Could you check a few things on this model? Use its own coordinates, in mm. A direction names the side the tool comes from. Give positions to 0.01 mm unless a question says otherwise; leave off trailing zeros. Loops run counter-clockwise (first coordinate to the right, second up) from the corner with the lowest first, then second, coordinate; pieces in that order, holes last. Notation, with made-up numbers: M -28.75,53.5 L 30.25,53.5 A21 ccw 30.25,87.5 Z; hole C 67.5,-13 d1. An arc over 180 degrees is marked long. Answer in a Markdown table with one row per item. Add a question column.
1. Thinking about a two-plate mould opening in Z: for faces 3 (the conical face through (-0.41, 22.857, 0.17)), 4 (the cylindrical face through (3.86, 92.6, 5.04)), 5 (the flat face through (-2, 187.82, 2)), 6 (the cylindrical face through (2.435, 11.466, -0.767)), which applies, released by +Z, released by -Z, zero draft, split by the parting line, or undercut?
2. I need wall thicknesses on line 1 along X through (y, z) = (101, -0.5); line 2 along Z through (x, y) = (-3.5, 45); line 3 along Z through (x, y) = (-0.75, 164.5). Which ranges of each line are inside material? Lowest first, please. Write a range as from..to.
3. Which directions (+Z, -Z, +X, -X, +Y, -Y) give clear straight access to the entire face, cutting with the end or side of a thin tool? Please do faces 1 (the flat face through (3, 0, -3)), 2 (the cylindrical face through (1.216, 178.676, -1.115)).
4. I'm going to push flat-ended pins straight in: pin 1 Ø3 at (x, y) = (-2, 79) entering from -Z; pin 2 Ø4 at (y, z) = (150, 2.5) entering from -X; pin 3 Ø4 at (x, z) = (0, 0) entering from -Y. Where does each tip first touch, or does it pass through?
5. If we section it at B-B on y = 155.5: List the corners of the cut face in (x, z) for me.
6. If we section it at A-A on y = 13: List the corners of the cut face in (x, z) for me, then the cut area to 3 significant figures.
```python
from build123d import *

# Parameters (mm, degrees)
SKETCH1_R                         = 6.35
BOSS_EXTRUDE1_DEPTH               = 187.8203
F_1_4_20_TAPPED_HOLE1_D           = 5.1054
F_1_4_20_TAPPED_HOLE1_DEPTH       = 21.59
F_1_4_20_TAPPED_HOLE1_CSINK_D     = 7.62
F_1_4_20_TAPPED_HOLE1_CSINK_ANGLE = 100
F_1_4_20_TAPPED_HOLE1_TIP         = 1.533816902
M4X0_7_TAPPED_HOLE1_D             = 3.3
M4X0_7_TAPPED_HOLE1_DEPTH         = 17.7292
M4X0_7_TAPPED_HOLE1_CSINK_D       = 4.05
M4X0_7_TAPPED_HOLE1_CSINK_ANGLE   = 100
M4X0_7_TAPPED_HOLE1_TIP           = 0.991420021


with BuildPart() as part:
    # Sketch1 → Boss-Extrude1 (new body)
    with BuildSketch(Plane(origin=(0, 0, 0), x_dir=(1, 0, 0), z_dir=(0, 1, 0))):
        with Locations(Location((0, 0, 0), (0, 0, 90))):
            Circle(SKETCH1_R)
    extrude(amount=BOSS_EXTRUDE1_DEPTH)

    # 1/4-20 Tapped Hole1
    with Locations(Plane(origin=(0, 0, 0), x_dir=(-1, 0, 0), z_dir=(0, -1, 0))):
        with Locations((0, 0)):
            CounterSinkHole(F_1_4_20_TAPPED_HOLE1_D / 2, F_1_4_20_TAPPED_HOLE1_CSINK_D / 2, depth=F_1_4_20_TAPPED_HOLE1_DEPTH, counter_sink_angle=F_1_4_20_TAPPED_HOLE1_CSINK_ANGLE)
            with Locations((0, 0, -(F_1_4_20_TAPPED_HOLE1_DEPTH + F_1_4_20_TAPPED_HOLE1_TIP / 2))):  # 118° drill point
                Cone(0, F_1_4_20_TAPPED_HOLE1_D / 2, F_1_4_20_TAPPED_HOLE1_TIP, mode=Mode.SUBTRACT)

    # M4x0.7 Tapped Hole1
    with Locations(Plane(origin=(0, 187.8203, 0), x_dir=(1, 0, 0), z_dir=(0, 1, 0))):
        with Locations((0, 0)):
            CounterSinkHole(M4X0_7_TAPPED_HOLE1_D / 2, M4X0_7_TAPPED_HOLE1_CSINK_D / 2, depth=M4X0_7_TAPPED_HOLE1_DEPTH, counter_sink_angle=M4X0_7_TAPPED_HOLE1_CSINK_ANGLE)
            with Locations((0, 0, -(M4X0_7_TAPPED_HOLE1_DEPTH + M4X0_7_TAPPED_HOLE1_TIP / 2))):  # 118° drill point
                Cone(0, M4X0_7_TAPPED_HOLE1_D / 2, M4X0_7_TAPPED_HOLE1_TIP, mode=Mode.SUBTRACT)


solid = part.part
```
Results:
| question | item | result |
|---|---|---|
| 1 | face 3 | undercut |
| 1 | face 4 | split by the parting line |
| 1 | face 5 | zero draft |
| 1 | face 6 | undercut |
| 2 | line 1 | -6.33..6.33 |
| 2 | line 2 | -5.3..5.3 |
| 2 | line 3 | -6.31..6.31 |
| 3 | face 1 | +Z, -Z, +X, -X, -Y |
| 3 | face 2 | +Y |
| 4 | pin 1 | z = -6.33 |
| 4 | pin 2 | x = -6.33 |
| 4 | pin 3 | y = 21.92 |
| 5 | outline | C 0,0 d12.7 |
| 6 | outline | C 0,0 d12.7; hole C 0,0 d5.11 |
| 6 | area | 106 mm2 |
